Autodesk Inventor part; units mm, degrees
ref_plane "YZ Plane" through (0, 0, 0) normal (1, 0, 0) x (0, 1, 0)
ref_plane "XZ Plane" through (0, 0, 0) normal (0, 1, 0) x (-1, 0, 0)
ref_plane "XY Plane" through (0, 0, 0) normal (0, 0, 1) x (1, 0, 0)
sketch "Sketch1" plane through (0, 0, 0) normal (0, 1, 0) x (-1, 0, 0)
  line L0 (0, 26.7471) -> (0, -19.6773)
  circle A0 centre (0, 0) radius 8
  line L1 (17.3205, 10) -> (100, -133.2051)
  line L2 (100, -133.2051) -> (0, -133.2051) construction
  line L3 (43.971, 0) -> (-53.4185, 0)
  line L4 (-17.3205, 10) -> (-100, -133.2051)
  line L5 (-100, -133.2051) -> (0, -133.2051) construction
  line L6 (-43.971, 0) -> (53.4185, 0)
  line L7 (100, -133.2051) -> (100, -193.2051)
  line L8 (100, -193.2051) -> (-100, -193.2051)
  line L9 (-100, -193.2051) -> (-100, -133.2051)
  arc A1 (17.3205, 10) -> (-17.3205, 10) centre (0, 0) ccw
  point P0 (0, 40)
  dimension "d0" = 16
  dimension "d2" = 100
  dimension "d3" = 80
  dimension "d4" = 60
  dimension "d5" = 60
  dimension "d6" = 20
extrude "Extrusion1" add sketch "Sketch1" along normal mid plane 384 contours A1 L1 L3 A0 L0 | L0 A0 L3 L4 A1 | L3 L1 L7 L8 L9 L4 A0
sketch "Sketch2" plane through (0, 0, 0) normal (1, 0, 0) x (0, 1, 0)
  line L0 (0, 110.6795) -> (0, -260.886)
  line L1 (-192, 20) -> (192, 20)
  line L2 (-182, 20) -> (-182, -90)
  line L3 (-182, -90) -> (-82.0296, -160)
  line L4 (-82.0296, -160) -> (0, -160)
  line L5 (-182, 20) -> (0, 20)
  line L6 (-192, 10) -> (-192, -133.2051)
  line L7 (182, 20) -> (182, -90)
  line L8 (182, -90) -> (82.0296, -160)
  line L9 (82.0296, -160) -> (0, -160)
  line L10 (182, 20) -> (0, 20)
  point P0 (0, 0)
  dimension "d9" = 10
  dimension "d10" = 180
  dimension "d11" = 110
  dimension "d12" = 145
extrude "Extrusion2" cut sketch "Sketch2" along normal through all both and the other way through all
sketch "Sketch3" plane through (0, 192, 0) normal (0, 1, 0) x (1, 0, 0)
  circle A0 centre (0, 0) radius 8
  line L0 (0, 0) -> (0, 264.7733)
  line L1 (-100, 193.2051) -> (100, 193.2051)
  line L2 (-82, 193.2051) -> (-62, 193.2051)
  line L3 (-62, 193.2051) -> (-62, 177.2051)
  line L4 (-62, 177.2051) -> (-82, 177.2051)
  line L5 (-82, 177.2051) -> (-82, 193.2051)
  line L6 (-100, 193.2051) -> (-100, 133.2051)
  line L7 (82, 193.2051) -> (62, 193.2051)
  line L8 (62, 193.2051) -> (62, 177.2051)
  line L9 (62, 177.2051) -> (82, 177.2051)
  line L10 (82, 177.2051) -> (82, 193.2051)
  dimension "d15" = 18
  dimension "d16" = 20
  dimension "d17" = 16
extrude "Extrusion3" cut sketch "Sketch3" against normal through all contours L3 L4 L5 L1 | L1 L10 L9 L8
properties part number "Y_axis"
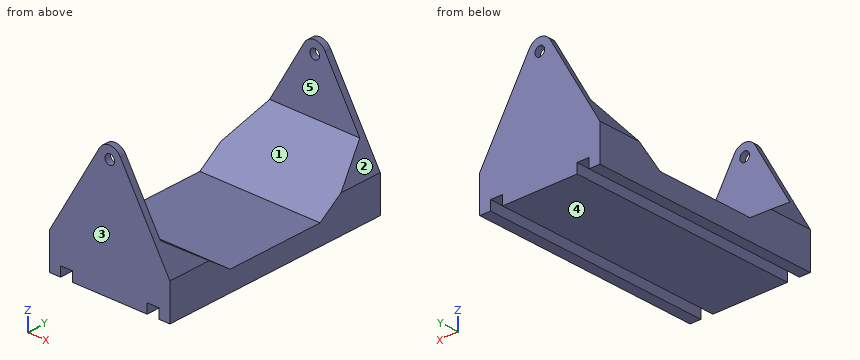
Design review of the part built by this model. Coordinates are the model's own, in mm. Face numbers are marked on the shaded views. A direction names the side the tool comes from. Coordinates: 2 decimals unless noted, no trailing zeros. Loops run counter-clockwise (first coordinate to the right, second up) from the corner with the lowest first, then second, coordinate; pieces in that order, holes last. Notation, with made-up numbers: (82.5, 54.5) -> (120.5, 54.5) arc R27 cw to (120.5, 86.5) -> close; hole circle Ø3 at (-5.75, 32). An arc over 180 degrees is marked (long way). Use a Markdown table: item, result. Add a question column.
Item 1: Wall thickness on L1, parallel to Y at x = 11, z = 5; L2, parallel to Y at x = 51, z = -144; L3, parallel to Z at x = 69.5, y = -28: over which ranges is each line inside the solid? List them lowest first. Write a range as from..to.
Item 2: We need section D-D, the plane z = 0. Write out the cut boundary in (x, y), and give its area (3 significant figures).
Item 3: Machinability: for the marked faces 4 and 5, which of the approach directions +Z, -Z, +X, -X, +Y, -Y give a long, thin tool a straight path to every point of the face, cutting with its end or side? Answer none if there is none.
Item 4: The part is to be moulded in two halves that separate along Y. For the marked faces 1, 2 and 3, say which applies: +Y half, -Y half, draft (parallel to the pull), parting line (faces both ways), or undercut.
Item 5: We need section B-B, the plane z = -95.5. Write out the cut boundary in (x, y).
Item 6: Clearance check with flat-ended pins moving along their axes: P1, Ø10, axis at x = 69.5, y = -13.5, coming from the -Z side; P2, Ø13, axis at x = 0, z = 0, coming from the -Y side. State where each tip first meets the part, or that it passes through.
Item 7: We need section C-C, the plane y = -55.5. Write out the cut boundary in (x, z).
Item 8: We need section A-A, the plane x = 0. Write out the cut boundary in (y, z), and give its area (3 significant figures).
Numbers:
| question | item | result |
|---|---|---|
| 1 | L1 | y = -192..-182, 182..192 |
| 1 | L2 | y = -192..-104.88, 104.88..192 |
| 1 | L3 | z = -177.21..-160 |
| 2 | outline | (-23.09, -192) -> (-8, -192) -> (-8, -182) -> (-23.09, -182) -> close; (-23.09, 182) -> (-8, 182) -> (-8, 192) -> (-23.09, 192) -> close; (8, -192) -> (23.09, -192) -> (23.09, -182) -> (8, -182) -> close; (8, 182) -> (23.09, 182) -> (23.09, 192) -> (8, 192) -> close |
| 2 | area | 604 mm^2 |
| 3 | face 4 | -Z, +X, -X, +Y, -Y |
| 3 | face 5 | +Z, +X, -X |
| 4 | face 1 | undercut |
| 4 | face 2 | draft |
| 4 | face 3 | -Y half |
| 5 | outline | (-78.23, -192) -> (78.23, -192) -> (78.23, -174.15) -> (-78.23, -174.15) -> close; (-78.23, 174.15) -> (78.23, 174.15) -> (78.23, 192) -> (-78.23, 192) -> close |
| 6 | P1 | stops at z = -177.21 |
| 6 | P2 | passes through |
| 7 | outline | (-100, -193.21) -> (-82, -193.21) -> (-82, -177.21) -> (-62, -177.21) -> (-62, -193.21) -> (62, -193.21) -> (62, -177.21) -> (82, -177.21) -> (82, -193.21) -> (100, -193.21) -> (100, -160) -> (-100, -160) -> close |
| 8 | outline | (-192, -193.21) -> (192, -193.21) -> (192, -8) -> (182, -8) -> (182, -90) -> (82.03, -160) -> (-82.03, -160) -> (-182, -90) -> (-182, -8) -> (-192, -8) -> close; (-192, 8) -> (-182, 8) -> (-182, 20) -> (-192, 20) -> close; (182, 8) -> (192, 8) -> (192, 20) -> (182, 20) -> close |
| 8 | area | 23,000 mm^2 |
